Can you work these out from the model? Positions are in its coordinate system, mm. Round coordinates to 2 decimals unless told otherwise and drop trailing zeros. Loops run counter-clockwise (first coordinate to the right, second up) from the corner with the lowest first, then second, coordinate; pieces in that order, holes last. Notation, with made-up numbers: (70.25, -0.75) -> (84.25, -0.75) arc R26 cw to (84.25, 35.25) -> close; hole circle Ø6 at (26.25, -33). An arc over 180 degrees is marked (long way). Use a Markdown table: item, result.
from build123d import *

# Parameters (mm, degrees)
F0_W     = 19.05
F0_H     = 37.4
F0_R     = 2
F1_DEPTH = 6.35
F2_R     = 4.1275
F3_DEPTH = 100
F4_SIZE  = 5


with BuildPart() as f1:
    # F0 (on Top) → F1 (new body)
    with BuildSketch(Plane.XY):
        Rectangle(F0_W, F0_H)
        with Locations((0, -12.7)):
            Circle(F0_R, mode=Mode.SUBTRACT)
        with Locations((0, 12.7)):
            Circle(F0_R, mode=Mode.SUBTRACT)
    extrude(amount=F1_DEPTH)

    # F2 (on face) → F3 (cut)
    with BuildSketch(Plane.YZ.offset(9.525)):
        with Locations((0, 6.75)):
            Circle(F2_R)
    extrude(amount=-F3_DEPTH, mode=Mode.SUBTRACT)

    # F4
    f4_edges = [f1.edges().sort_by_distance(p)[0] for p in [
        (9.525, -18.7, 3.175),
        (-9.525, -18.7, 3.175),
        (-9.525, 18.7, 3.175),
        (9.525, 18.7, 3.175),
    ]]
    chamfer(f4_edges, length=F4_SIZE)


solid = f1.part
1. Will these pins go through, and if not, where does the flat tip stop? pin 1 Ø1 at (x, y) = (1, 2) entering from +Z; pin 2 Ø3 at (x, y) = (0, 12.7) entering from -Z.
Answer sheet:
| item | result |
|---|---|
| pin 1 | stops at z = 3.47 |
| pin 2 | passes through |
2. I want a section at B-B (y = -12.7). Please give me the cut outline in (x, z) (3 decimals).
Answer sheet:
| item | result |
|---|---|
| outline | (-9.525, 0) -> (-2, 0) -> (-2, 6.35) -> (-9.525, 6.35) -> close; (2, 0) -> (9.525, 0) -> (9.525, 6.35) -> (2, 6.35) -> close |
3. I need wall thicknesses on line 1 (Y direction, x = 0, z = 1.75); line 2 (Y direction, x = 0, z = 5); line 3 (Y direction, x = -5.75, z = 5.25) (3 decimals). Which ranges of each line are inside material? Lowest first, please.
Answer sheet:
| item | result |
|---|---|
| line 1 | y = -18.7 to -14.7, -10.7 to 10.7, 14.7 to 18.7 |
| line 2 | y = -18.7 to -14.7, -10.7 to -3.74, 3.74 to 10.7, 14.7 to 18.7 |
| line 3 | y = -17.475 to -3.845, 3.845 to 17.475 |
4. I want a section at C-C (x = 0). State how many separate pieces and enclosed holes the cut face has, plus the area to 3 significant figures.
Answer sheet:
| item | result |
|---|---|
| separate pieces | 3 |
| enclosed holes | 0 |
| area | 163 mm² |
5. If we mould it in two halves opening along Y, with no side actions, what happens to faces 1 (the cylindrical face through (0.133, -0.085, 2.623)), 2 (the flat face through (0, -10, 6.35)), 3 (the flat face through (7.06, -16.165, 3.131)), 4 (the flat face through (0, 18.7, 3))? For each: +Y half, -Y half, draft (parallel to the pull), parting line (faces both ways), or undercut.
Answer sheet:
| item | result |
|---|---|
| face 1 | undercut |
| face 2 | draft |
| face 3 | -Y half |
| face 4 | +Y half |
6. I want a section at A-A (z = 3). Please give me the cut outline in (x, y) (3 decimals), plus the area to 3 significant figures.
Answer sheet:
| item | result |
|---|---|
| outline | (-9.525, -13.7) -> (-4.525, -18.7) -> (4.525, -18.7) -> (9.525, -13.7) -> (9.525, -1.724) -> (-9.525, -1.724) -> close; (-9.525, 1.724) -> (9.525, 1.724) -> (9.525, 13.7) -> (4.525, 18.7) -> (-4.525, 18.7) -> (-9.525, 13.7) -> close; hole circle Ø4 at (0, -12.7); hole circle Ø4 at (0, 12.7) |
| area | 572 mm² |
7. I want a section at D-D (z = 5.25). Please give me the cut outline in (x, y) (3 decimals).
Answer sheet:
| item | result |
|---|---|
| outline | (-9.525, -13.7) -> (-4.525, -18.7) -> (4.525, -18.7) -> (9.525, -13.7) -> (9.525, -3.845) -> (-9.525, -3.845) -> close; (-9.525, 3.845) -> (9.525, 3.845) -> (9.525, 13.7) -> (4.525, 18.7) -> (-4.525, 18.7) -> (-9.525, 13.7) -> close; hole circle Ø4 at (0, -12.7); hole circle Ø4 at (0, 12.7) |
